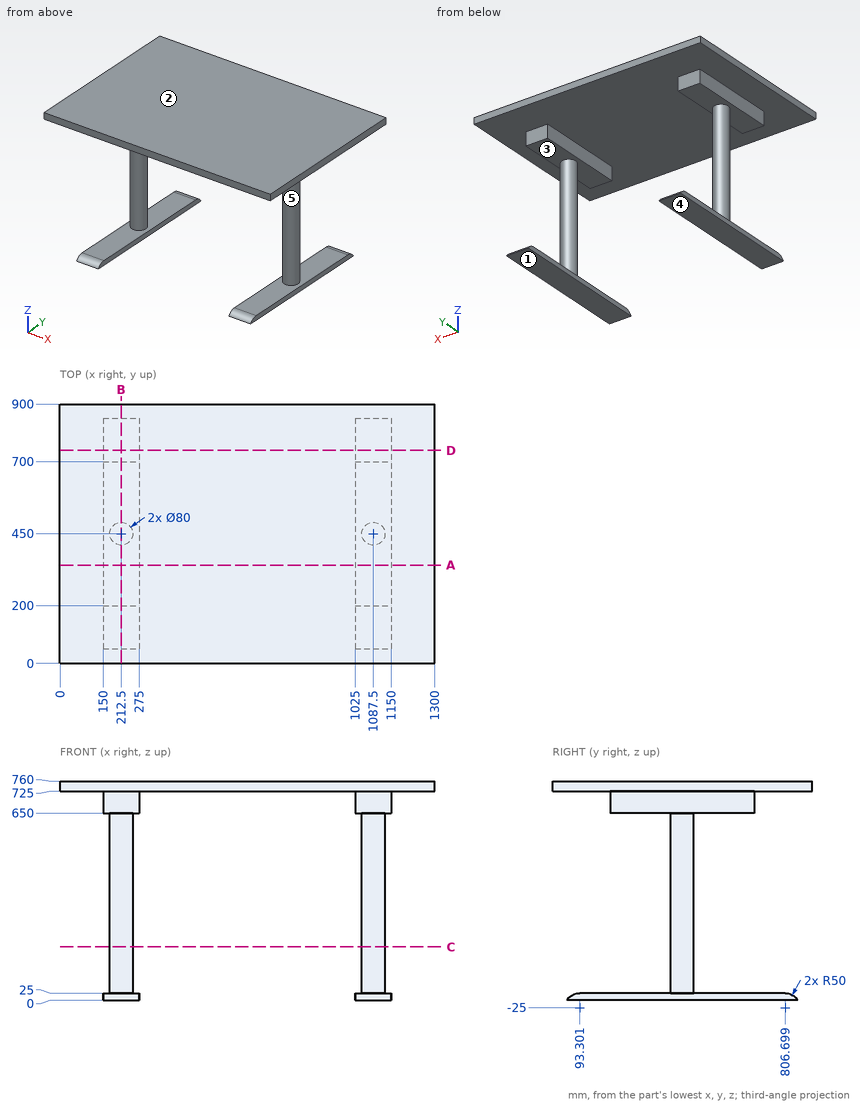
Study the drawing (mm; zero at the part's minimum x, y, z) and answer. A direction names the side the tool comes from. Give positions to 0.01 mm unless a question says otherwise; leave off trailing zeros. Write each loop counter-clockwise with the first axis right and the second up, starting at its lowest first coordinate (ties: lowest second). Pieces come first, ordered by that corner, then holes. Notation, with made-up numbers: M 76.5,34 L 117.5,34 A10 ccw 117.5,50 Z; hole C -35,10 d11. An arc over 180 degrees is marked long. Put each result on its own line as item: value. Start each with the question number.
1. The part is cut by section A-A, the plane y = 341. Give the vertices of the cut face in (x, z).
2. For a pull along Z with two mould halves and no side action, classify the marked faces 1, 2 and 3 as released by +Z, released by -Z, zero draft, split by the parting line, or undercut.
3. The part is cut by section B-B, the plane x = 212.5. Give the vertices of the cut face in (y, z).
4. Each of these flat-tipped pins is pushed along its axis until it touches: pin 1 Ø7.5 at (y, z) = (610, 18.5) entering from +X; pin 2 Ø1.5 at (x, y) = (1011, 247.5) entering from -Z; pin 3 Ø12 at (x, y) = (212.5, 634) entering from -Z; pin 4 Ø7.5 at (y, z) = (340.5, 13) entering from -X. Where does it stop, or does it pass through?
5. Consider line 1 along Z through (x, y) = (186, 342); line 2 along Z through (x, y) = (368, 333); line 3 along Z through (x, y) = (1047, 726). Determine where each line is inside the solid, lowest interval first.
6. The part is cut by section D-D, the plane y = 739. Give the vertices of the cut face in (x, z).
7. Which of the six approach directions +Z, -Z, +X, -X, +Y, -Y give full straight-line access (tool end or side, diameter ignored) to the marked faces 4 and 5?
8. The part is cut by section C-C, the plane z = 186. Give the vertices of the cut face in (x, y), and give its area (3 significant figures).
Final values:
1. outline: M 0,725 L 150,725 L 150,650 L 275,650 L 275,725 L 1025,725 L 1025,650 L 1150,650 L 1150,725 L 1300,725 L 1300,760 L 0,760 Z; M 150,0 L 275,0 L 275,25 L 150,25 Z; M 1025,0 L 1150,0 L 1150,25 L 1025,25 Z
2. face 1: released by -Z
2. face 2: released by +Z
2. face 3: undercut
3. outline: M 0,725 L 200,725 L 200,650 L 410,650 L 410,25 L 93.3,25 A50 ccw 50,0 L 850,0 A50 ccw 806.7,25 L 490,25 L 490,650 L 700,650 L 700,725 L 900,725 L 900,760 L 0,760 Z
4. pin 1: stops at x = 1150
4. pin 2: stops at z = 725
4. pin 3: stops at z = 0
4. pin 4: stops at x = 150
5. line 1: z = 0 to 25, 650 to 760
5. line 2: z = 725 to 760
5. line 3: z = 0 to 25, 725 to 760
6. outline: M 0,725 L 1300,725 L 1300,760 L 0,760 Z; M 150,0 L 275,0 L 275,25 L 150,25 Z; M 1025,0 L 1150,0 L 1150,25 L 1025,25 Z
7. face 4: -Z, +X, -X, +Y, -Y
7. face 5: none
8. outline: C 212.5,450 d80; C 1087.5,450 d80
8. area: 10,100 mm²
